The drawing under review shows one solid part. Ordinate dimensions are in mm from its lowest x, y, z. Coordinates: 2 decimals unless noted, no trailing zeros. Write each loop counter-clockwise with the first axis right and the second up, starting at its lowest first coordinate (ties: lowest second). Pieces come first, ordered by that corner, then holes. Notation, with made-up numbers: (35.5, -25) -> (59.5, -25) arc R21 cw to (59.5, -7) -> close; hole circle Ø1 at (3, 34). An arc over 180 degrees is marked (long way). One line per item, written item: value. Start each with the question number.
1) For probe 1 along Y at (x, z) = (76.2, 1); probe 2 along X at (y, z) = (83, 1.85) (1 decimal); probe 3 along X at (y, z) = (58, 1.4) (1 decimal), list the stretches that pass through material, from the lowest coordinate up. Write a range as from..to.
2) For pin 1 Ø1.5 at (x, z) = (63.5, 1.5) entering from +Y; pin 2 Ø1 at (y, z) = (59.5, 2) entering from +X; pin 3 Ø1.5 at (x, z) = (131.5, 1.5) entering from -Y (1 decimal), all flat-tipped, find the tip position at first contact; note any pin that passes through.
3) Add section D-D (x = 132.5). State the section outline as (y, z) points.
4) Add section A-A (x = 76.2). State the section outline as (y, z) points.
5) Add section C-C (z = 1.7). State the section outline as (x, y) points, and give its area (3 significant figures).
6) Add section B-B (y = 76.2). State the section outline as (x, z) points.
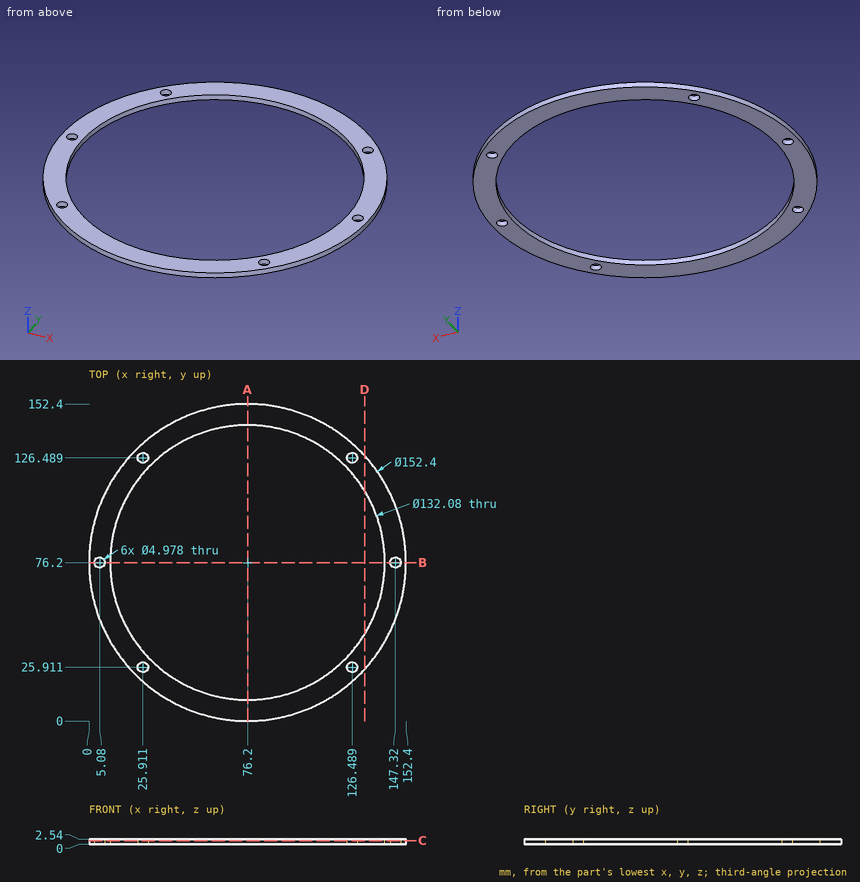
Numbers:
1. probe 1: 0..10.16, 142.24..152.4
1. probe 2: 0.3..10.5, 141.9..152.1
1. probe 3: 2.2..12.7, 139.7..150.2
2. pin 1: y = 151.46
2. pin 2: x = 150.66
2. pin 3: y = 23
3. outline: (24.85, 0) -> (41.68, 0) -> (41.68, 2.54) -> (24.85, 2.54) -> close; (110.72, 0) -> (127.55, 0) -> (127.55, 2.54) -> (110.72, 2.54) -> close
4. outline: (0, 0) -> (10.16, 0) -> (10.16, 2.54) -> (0, 2.54) -> close; (142.24, 0) -> (152.4, 0) -> (152.4, 2.54) -> (142.24, 2.54) -> close
5. outline: circle Ø152.4 at (76.2, 76.2); hole circle Ø4.98 at (5.08, 76.2); hole circle Ø132.08 at (76.2, 76.2); hole circle Ø4.98 at (25.91, 25.91); hole circle Ø4.98 at (25.91, 126.49); hole circle Ø4.98 at (126.49, 25.91); hole circle Ø4.98 at (126.49, 126.49); hole circle Ø4.98 at (147.32, 76.2)
5. area: 4,420 mm²
6. outline: (0, 0) -> (2.59, 0) -> (2.59, 2.54) -> (0, 2.54) -> close; (7.57, 0) -> (10.16, 0) -> (10.16, 2.54) -> (7.57, 2.54) -> close; (142.24, 0) -> (144.83, 0) -> (144.83, 2.54) -> (142.24, 2.54) -> close; (149.81, 0) -> (152.4, 0) -> (152.4, 2.54) -> (149.81, 2.54) -> close
